```python
from build123d import *

# Parameters (mm, degrees)
SKETCH_1_R      = 4
EXTRUDE_1_DEPTH = 50


with BuildPart() as part:
    # 草图1 → 凸台-拉伸1 (new, symmetric)
    with BuildSketch(Plane.XY):
        Circle(SKETCH_1_R)
    extrude(amount=EXTRUDE_1_DEPTH, both=True)

    # 草图3 → M5 螺纹孔1 (revolve, cut)
    with BuildSketch(Plane(origin=(0, 0, 50), x_dir=(0, -1, 0), z_dir=(1, 0, 0))):
        Polygon((0, 0), (0, 13.6618073), (2.1, 12.4), (2.1, 0), align=None)
    hole_wizard_m5_1 = revolve(axis=Axis((0, 0, 56.35), (0, 0, -1)), mode=Mode.SUBTRACT)

    # 镜向1: M5 螺纹孔1 across plane
    add(hole_wizard_m5_1.mirror(Plane.XY), mode=Mode.SUBTRACT)


solid = part.part
```
The listing builds one solid part. Answer for the finished solid, in the listing's coordinates (mm). A direction names the side the tool comes from. Coordinates: 2 decimals unless noted, no trailing zeros. Write each loop counter-clockwise with the first axis right and the second up, starting at its lowest first coordinate (ties: lowest second). Pieces come first, ordered by that corner, then holes. Notation, with made-up numbers: (69, 51.25) -> (95, 51.25) arc R8 cw to (95, 58.25) -> close; hole circle Ø9 at (39, 63.5). An arc over 180 degrees is marked (long way). Write each question's results on one line, items separated by ' | '. Start each with the question number.
1) A tool of negligible diameter and unlimited length cuts with its end or side. For faces 1 (the conical face through (-0.11, -0.35, 36.56)), 2 (the cylindrical face through (-0.631, -2.003, -43.887)), from which of +Z, -Z, +X, -X, +Y, -Y can it reach the whole face along a straight path? Write none if from no direction.
2) A cutting plane is placed at A-A (z = -43.5). Determine the outline of the cut face in (x, y), then the cut area to 3 significant figures.
3) A cutting plane is placed at B-B (z = -29.5). Determine the outline of the cut face in (x, y), then the cut area to 3 significant figures.
4) For a pull along X with two mould halves and no side action, classify faces 3 (the cylindrical face through (-0.631, -2.003, 43.887)), 4 (the cylindrical face through (-0.867, -3.905, 0.7)), 5 (the flat face through (2, -2, -50)) as +X half, -X half, draft (parallel to the pull), parting line (faces both ways), or undercut.
5) Straight lines are drawn through the part: probe 1 along Y at (x, z) = (0, -47); probe 2 along Y at (x, z) = (1.25, 25); probe 3 along Y at (x, z) = (3, -36). For each, find the intervals that lie inside material, in ascending order.
6) Flat-ended cylindrical pins translate along their axes: pin 1 Ø2.5 at (x, y) = (0, 0) entering from -Z; pin 2 Ø4 at (x, y) = (0, 2) entering from -Z. Find the tip coordinate at first contact, or state that the pin passes through.
Values follow:
1) face 1: +Z | face 2: -Z
2) outline: circle Ø8 at (0, 0); hole circle Ø4.2 at (0, 0) | area: 36.4 mm²
3) outline: circle Ø8 at (0, 0) | area: 50.3 mm²
4) face 3: undercut | face 4: parting line | face 5: draft
5) probe 1: -4 to -2.1, 2.1 to 4 | probe 2: -3.8 to 3.8 | probe 3: -2.65 to 2.65
6) pin 1: z = -37.09 | pin 2: z = -50
